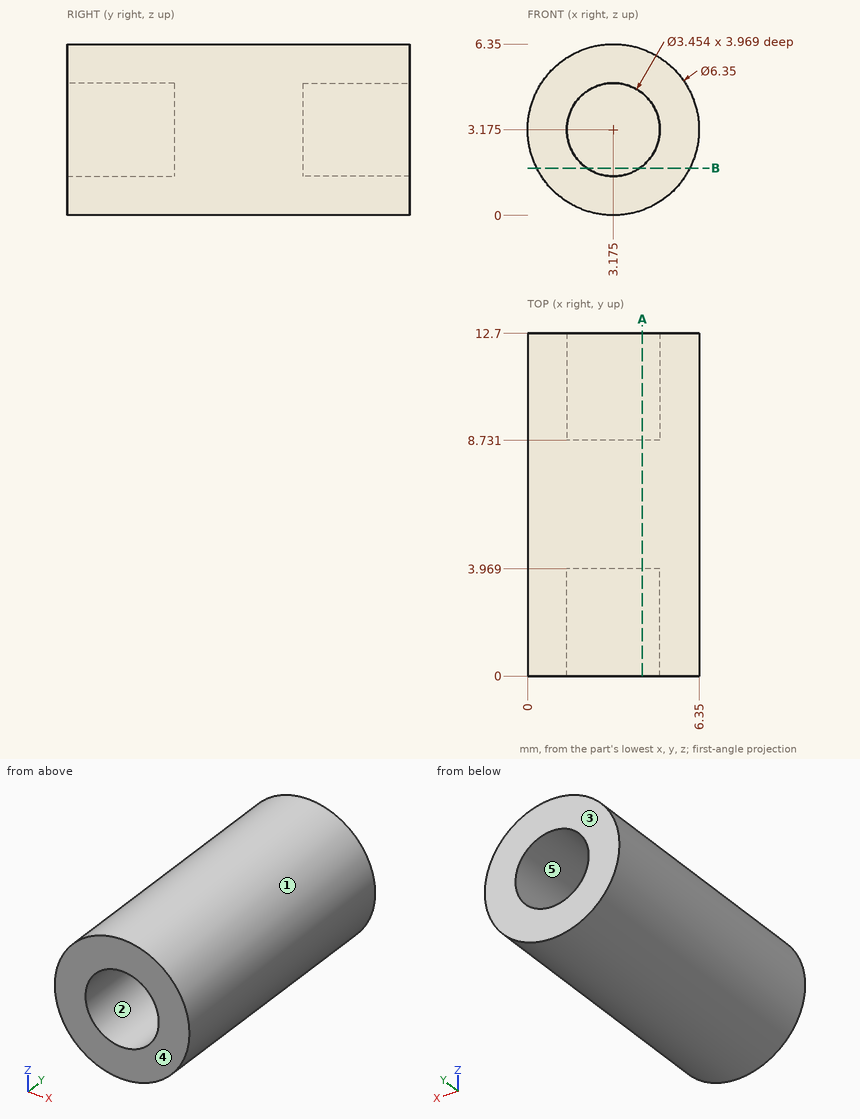
Print and shaded views of the part. All mm, measured from the part's lowest x, y and z. A direction names the side the tool comes from. Give positions to 0.01 mm unless a question says otherwise; leave off trailing zeros. Loops run counter-clockwise (first coordinate to the right, second up) from the corner with the lowest first, then second, coordinate; pieces in that order, holes last. Notation, with made-up numbers: M -1.5,57 L 31.5,57 A8 ccw 31.5,69 Z; hole C -26.5,76 d1. An arc over 180 degrees is marked long. Write each question's results on one line, items separated by ' | '.
Q1. Mould opens along Z. For the marked faces 1, 2 and 3 say: pulls with the +Z half, pulls with the -Z half, needs draft (parallel to the pull), parting line crosses it, or undercut.
Geometry check:
face 1: parting line crosses it | face 2: undercut | face 3: needs draft
Q2. Band-saw the part on B-B on z = 1.75. Write the cut outline in (x, y).
Geometry check:
outline: M 0.34,0 L 2.2,0 L 2.2,3.97 L 4.15,3.97 L 4.15,0 L 6.01,0 L 6.01,12.7 L 4.15,12.7 L 4.15,8.73 L 2.2,8.73 L 2.2,12.7 L 0.34,12.7 Z
Q3. Flat gauge pins, fed straight in: P1, Ø1.5, axis at x = 1, y = 3.5, coming from the +Z side; P2, Ø1, axis at x = 3.5, z = 3.5, coming from the -Y side; P3, Ø1.5, axis at y = 2, z = 4.5, coming from the -X side. Where does each tip first touch, or does it go through?
Geometry check:
P1: stops at z = 6.01 | P2: stops at y = 3.97 | P3: stops at x = 0.05
Q4. Band-saw the part on A-A on x = 4.25. Write the cut outline in (y, z).
Geometry check:
outline: M 0,0.19 L 12.7,0.19 L 12.7,1.82 L 8.73,1.82 L 8.73,4.53 L 12.7,4.53 L 12.7,6.16 L 0,6.16 L 0,4.53 L 3.97,4.53 L 3.97,1.82 L 0,1.82 Z
Q5. Which spindle directions (+Z, -Z, +X, -X, +Y, -Y) get a long thin tool onto all of the face, cutting with end or side? Do the marked faces 4 and 5. Say none if no direction does.
Geometry check:
face 4: +Z, -Z, +X, -X, -Y | face 5: +Y
Q6. Probe probe 1 along X at (y, z) = (11.25, 3.25); probe 2 along Z at (x, y) = (3, 10.25) (1 decimal); probe 3 along X at (y, z) = (11.5, 2.25) (1 decimal). List the from-to ranges inside material, lowest first.
Geometry check:
probe 1: x = 0 to 1.45, 4.9 to 6.35 | probe 2: z = 0 to 1.5, 4.9 to 6.3 | probe 3: x = 0.1 to 1.7, 4.6 to 6.2
